Work out the finished part from the listing and answer in its coordinate system (mm). A direction names the side the tool comes from. Coordinates: 2 decimals unless noted, no trailing zeros. Write each loop counter-clockwise with the first axis right and the second up, starting at its lowest first coordinate (ties: lowest second). Pieces come first, ordered by that corner, then holes. Notation, with made-up numbers: M 25,65.25 L 57,65.25 A18 cw 57,81.25 Z; hole C -31,-27.75 d1. An arc over 180 degrees is marked long. Answer as CSV lines item,"result". Start each with the question number.
(1) The mould has two halves that part along Y. Classify faces 6 (the cylindrical face through (36.444, 55.404, 6.409)), 7 (the flat face through (16, 1, 0)), 8 (the cylindrical face through (36.36, -55.38, 6.41)), 9 (the cylindrical face through (-48.234, 45.511, 6.409)): released by +Y, released by -Y, zero draft, split by the parting line, or undercut.
(2) Find the intervals of material crossed by L1, parallel to Y at x = -53.5, z = 11.75; L2, parallel to X at y = -65, z = 8.25; L3, parallel to X at y = 56, z = 9, in increasing order. Write a range as [from, to].
(3) For faces 1 (the flat face through (-17.42, -70, 6.41)), 2 (the flat face through (0, 0, 2)), 3 (the cylindrical face through (-29.78, -59.18, 6.41)), 4 (the flat face through (51.909, -50.084, 6.409)), 5 (the flat face through (-51.909, 50.084, 6.409)), determine the directions among +Z, -Z, +X, -X, +Y, -Y from which every point of the face is accessible in a straight line to the end or side of a thin tool.
(4) A cutting plane is placed at A-A on x = 0. Give the vertices of the cut face in (y, z).
(5) A cutting plane is placed at B-B on z = -3. Give the vertices of the cut face in (x, y), then the cut area to 3 significant figures.
(6) Flat-ended cylindrical pins translate along their axes: P1, Ø3, axis at x = -21, y = 3, coming from the +Z side; P2, Ø2, axis at y = 0, z = 8.5, coming from the -X side; P3, Ø0.9, axis at x = 5, y = -7.5, coming from the -Z side; P4, Ø1, axis at y = -17.5, z = -1.5, coming from the +X side. Find the tip coordinate at first contact, or state that the pin passes through.
from build123d import *

# Parameters (mm, degrees)
F0_R     = 62.5
F0_R_2   = 12.7
F0_R_3   = 1.5
F0_R_4   = 4
F1_DEPTH = 3
F2_DEPTH = 13
F3_DEPTH = 9.5
F4_DEPTH = 2


with BuildPart() as f1:
    # F0 (on Top) → F1 (new body)
    with BuildSketch(Plane.XY):
        Circle(F0_R)
        Circle(F0_R_2, mode=Mode.SUBTRACT)
        Circle(F0_R_2)
        with Locations((-4.75, -8.227241)):
            Circle(F0_R_3, mode=Mode.SUBTRACT)
        with Locations((4.75, -8.227241)):
            Circle(F0_R_3, mode=Mode.SUBTRACT)
        with Locations((-9.5, 0)):
            Circle(F0_R_3, mode=Mode.SUBTRACT)
        with Locations((-4.75, 8.227241)):
            Circle(F0_R_3, mode=Mode.SUBTRACT)
        Circle(F0_R_4, mode=Mode.SUBTRACT)
        with Locations((4.75, 8.227241)):
            Circle(F0_R_3, mode=Mode.SUBTRACT)
        with Locations((9.5, 0)):
            Circle(F0_R_3, mode=Mode.SUBTRACT)
        with Locations((9.5, 0)):
            Circle(F0_R_3)
        with Locations((4.75, 8.227241)):
            Circle(F0_R_3)
        with Locations((-4.75, 8.227241)):
            Circle(F0_R_3)
        with Locations((-9.5, 0)):
            Circle(F0_R_3)
        with Locations((-4.75, -8.227241)):
            Circle(F0_R_3)
        with Locations((4.75, -8.227241)):
            Circle(F0_R_3)
    extrude(amount=F1_DEPTH)

    # F0 (on Top) → F2 (join)
    with BuildSketch(Plane.XY):
        with BuildLine():
            Line((69, 5), (74.833148, 5))
            ThreePointArc((74.833148, 5), (73.860581, 13.023613), (72.030257, 20.895981))
            Line((72.030257, 20.895981), (66.548892, 18.900927))
            ThreePointArc((66.548892, 18.900927), (63.490338, 19.034466), (61.42204, 21.291617))
            Line((61.42204, 21.291617), (60.738, 23.171002))
            ThreePointArc((60.738, 23.171002), (60.87154, 26.229556), (63.12869, 28.297853))
            Line((63.12869, 28.297853), (68.610056, 30.292907))
            ThreePointArc((68.610056, 30.292907), (64.951905, 37.5), (60.539455, 44.271598))
            Line((60.539455, 44.271598), (56.071005, 40.522123))
            ThreePointArc((56.071005, 40.522123), (53.151231, 39.601522), (50.435676, 41.01515))
            Line((50.435676, 41.01515), (49.150101, 42.547239))
            ThreePointArc((49.150101, 42.547239), (48.2295, 45.467012), (49.643129, 48.182567))
            Line((49.643129, 48.182567), (54.111579, 51.932042))
            ThreePointArc((54.111579, 51.932042), (48.209071, 57.453333), (41.746701, 62.307407))
            Line((41.746701, 62.307407), (38.830127, 57.255753))
            ThreePointArc((38.830127, 57.255753), (36.401302, 55.39205), (33.366025, 55.791651))
            Line((33.366025, 55.791651), (31.633975, 56.791651))
            ThreePointArc((31.633975, 56.791651), (29.770271, 59.220477), (30.169873, 62.255753))
            Line((30.169873, 62.255753), (33.086447, 67.307407))
            ThreePointArc((33.086447, 67.307407), (25.651511, 70.476947), (17.918678, 72.828023))
            Line((17.918678, 72.828023), (16.905763, 67.083494))
            ThreePointArc((16.905763, 67.083494), (15.260838, 64.501479), (12.271939, 63.838856))
            Line((12.271939, 63.838856), (10.302324, 64.186152))
            ThreePointArc((10.302324, 64.186152), (7.720308, 65.831077), (7.057685, 68.819976))
            Line((7.057685, 68.819976), (8.070601, 74.564505))
            ThreePointArc((8.070601, 74.564505), (0, 75), (-8.070601, 74.564505))
            Line((-8.070601, 74.564505), (-7.057685, 68.819976))
            ThreePointArc((-7.057685, 68.819976), (-7.720308, 65.831077), (-10.302324, 64.186152))
            Line((-10.302324, 64.186152), (-12.271939, 63.838856))
            ThreePointArc((-12.271939, 63.838856), (-15.260838, 64.501479), (-16.905763, 67.083494))
            Line((-16.905763, 67.083494), (-17.918678, 72.828023))
            ThreePointArc((-17.918678, 72.828023), (-25.651511, 70.476947), (-33.086447, 67.307407))
            Line((-33.086447, 67.307407), (-30.169873, 62.255753))
            ThreePointArc((-30.169873, 62.255753), (-29.770271, 59.220477), (-31.633975, 56.791651))
            Line((-31.633975, 56.791651), (-33.366025, 55.791651))
            ThreePointArc((-33.366025, 55.791651), (-36.401302, 55.39205), (-38.830127, 57.255753))
            Line((-38.830127, 57.255753), (-41.746701, 62.307407))
            ThreePointArc((-41.746701, 62.307407), (-48.209071, 57.453333), (-54.111579, 51.932042))
            Line((-54.111579, 51.932042), (-49.643129, 48.182567))
            ThreePointArc((-49.643129, 48.182567), (-48.2295, 45.467012), (-49.150101, 42.547239))
            Line((-49.150101, 42.547239), (-50.435676, 41.01515))
            ThreePointArc((-50.435676, 41.01515), (-53.151231, 39.601522), (-56.071005, 40.522123))
            Line((-56.071005, 40.522123), (-60.539455, 44.271598))
            ThreePointArc((-60.539455, 44.271598), (-64.951905, 37.5), (-68.610056, 30.292907))
            Line((-68.610056, 30.292907), (-63.12869, 28.297853))
            ThreePointArc((-63.12869, 28.297853), (-60.87154, 26.229556), (-60.738, 23.171002))
            Line((-60.738, 23.171002), (-61.42204, 21.291617))
            ThreePointArc((-61.42204, 21.291617), (-63.490338, 19.034466), (-66.548892, 18.900927))
            Line((-66.548892, 18.900927), (-72.030257, 20.895981))
            ThreePointArc((-72.030257, 20.895981), (-73.860581, 13.023613), (-74.833148, 5))
            Line((-74.833148, 5), (-69, 5))
            ThreePointArc((-69, 5), (-66.171573, 3.828427), (-65, 1))
            Line((-65, 1), (-65, -1))
            ThreePointArc((-65, -1), (-66.171573, -3.828427), (-69, -5))
            Line((-69, -5), (-74.833148, -5))
            ThreePointArc((-74.833148, -5), (-73.860581, -13.023613), (-72.030257, -20.895981))
            Line((-72.030257, -20.895981), (-66.548892, -18.900927))
            ThreePointArc((-66.548892, -18.900927), (-63.490338, -19.034466), (-61.42204, -21.291617))
            Line((-61.42204, -21.291617), (-60.738, -23.171002))
            ThreePointArc((-60.738, -23.171002), (-60.87154, -26.229556), (-63.12869, -28.297853))
            Line((-63.12869, -28.297853), (-68.610056, -30.292907))
            ThreePointArc((-68.610056, -30.292907), (-64.951905, -37.5), (-60.539455, -44.271598))
            Line((-60.539455, -44.271598), (-56.071005, -40.522123))
            ThreePointArc((-56.071005, -40.522123), (-53.151231, -39.601522), (-50.435676, -41.01515))
            Line((-50.435676, -41.01515), (-49.150101, -42.547239))
            ThreePointArc((-49.150101, -42.547239), (-48.2295, -45.467012), (-49.643129, -48.182567))
            Line((-49.643129, -48.182567), (-54.111579, -51.932042))
            ThreePointArc((-54.111579, -51.932042), (-48.209071, -57.453333), (-41.746701, -62.307407))
            Line((-41.746701, -62.307407), (-38.830127, -57.255753))
            ThreePointArc((-38.830127, -57.255753), (-36.401302, -55.39205), (-33.366025, -55.791651))
            Line((-33.366025, -55.791651), (-31.633975, -56.791651))
            ThreePointArc((-31.633975, -56.791651), (-29.770271, -59.220477), (-30.169873, -62.255753))
            Line((-30.169873, -62.255753), (-33.086447, -67.307407))
            ThreePointArc((-33.086447, -67.307407), (-25.651511, -70.476947), (-17.918678, -72.828023))
            Line((-17.918678, -72.828023), (-16.905763, -67.083494))
            ThreePointArc((-16.905763, -67.083494), (-15.260838, -64.501479), (-12.271939, -63.838856))
            Line((-12.271939, -63.838856), (-10.302324, -64.186152))
            ThreePointArc((-10.302324, -64.186152), (-7.720308, -65.831077), (-7.057685, -68.819976))
            Line((-7.057685, -68.819976), (-8.070601, -74.564505))
            ThreePointArc((-8.070601, -74.564505), (0, -75), (8.070601, -74.564505))
            Line((8.070601, -74.564505), (7.057685, -68.819976))
            ThreePointArc((7.057685, -68.819976), (7.720308, -65.831077), (10.302324, -64.186152))
            Line((10.302324, -64.186152), (12.271939, -63.838856))
            ThreePointArc((12.271939, -63.838856), (15.260838, -64.501479), (16.905763, -67.083494))
            Line((16.905763, -67.083494), (17.918678, -72.828023))
            ThreePointArc((17.918678, -72.828023), (25.651511, -70.476947), (33.086447, -67.307407))
            Line((33.086447, -67.307407), (30.169873, -62.255753))
            ThreePointArc((30.169873, -62.255753), (29.770271, -59.220477), (31.633975, -56.791651))
            Line((31.633975, -56.791651), (33.366025, -55.791651))
            ThreePointArc((33.366025, -55.791651), (36.401302, -55.39205), (38.830127, -57.255753))
            Line((38.830127, -57.255753), (41.746701, -62.307407))
            ThreePointArc((41.746701, -62.307407), (48.209071, -57.453333), (54.111579, -51.932042))
            Line((54.111579, -51.932042), (49.643129, -48.182567))
            ThreePointArc((49.643129, -48.182567), (48.2295, -45.467012), (49.150101, -42.547239))
            Line((49.150101, -42.547239), (50.435676, -41.01515))
            ThreePointArc((50.435676, -41.01515), (53.151231, -39.601522), (56.071005, -40.522123))
            Line((56.071005, -40.522123), (60.539455, -44.271598))
            ThreePointArc((60.539455, -44.271598), (64.951905, -37.5), (68.610056, -30.292907))
            Line((68.610056, -30.292907), (63.12869, -28.297853))
            ThreePointArc((63.12869, -28.297853), (60.87154, -26.229556), (60.738, -23.171002))
            Line((60.738, -23.171002), (61.42204, -21.291617))
            ThreePointArc((61.42204, -21.291617), (63.490338, -19.034466), (66.548892, -18.900927))
            Line((66.548892, -18.900927), (72.030257, -20.895981))
            ThreePointArc((72.030257, -20.895981), (73.860581, -13.023613), (74.833148, -5))
            Line((74.833148, -5), (69, -5))
            ThreePointArc((69, -5), (66.171573, -3.828427), (65, -1))
            Line((65, -1), (65, 1))
            ThreePointArc((65, 1), (66.171573, 3.828427), (69, 5))
        make_face()
        Circle(F0_R, mode=Mode.SUBTRACT)
    extrude(amount=F2_DEPTH)

    # F0 (on Top) → F3 (join)
    with BuildSketch(Plane.XY):
        Circle(F0_R_2)
        with Locations((-4.75, -8.227241)):
            Circle(F0_R_3, mode=Mode.SUBTRACT)
        with Locations((4.75, -8.227241)):
            Circle(F0_R_3, mode=Mode.SUBTRACT)
        with Locations((-9.5, 0)):
            Circle(F0_R_3, mode=Mode.SUBTRACT)
        with Locations((-4.75, 8.227241)):
            Circle(F0_R_3, mode=Mode.SUBTRACT)
        Circle(F0_R_4, mode=Mode.SUBTRACT)
        with Locations((4.75, 8.227241)):
            Circle(F0_R_3, mode=Mode.SUBTRACT)
        with Locations((9.5, 0)):
            Circle(F0_R_3, mode=Mode.SUBTRACT)
        with Locations((-4.75, 8.227241)):
            Circle(F0_R_3)
        with Locations((9.5, 0)):
            Circle(F0_R_3)
        with Locations((-4.75, -8.227241)):
            Circle(F0_R_3)
    extrude(amount=-F3_DEPTH)

    # F0 (on Top) → F4 (join)
    with BuildSketch(Plane.XY):
        Circle(F0_R_4)
    extrude(amount=F4_DEPTH)


solid = f1.part
Here are the results:
1,face 6,"released by +Y"
1,face 7,"zero draft"
1,face 8,"released by -Y"
1,face 9,"undercut"
2,L1,"y = [-52.56, -51.42], [-39.59, -32.31], [32.31, 39.59], [51.42, 52.56]"
2,L2,"x = [-31.75, -15.84], [-8.5, 8.5], [15.84, 31.75]"
2,L3,"x = [-49.89, -37.69], [-33.01, -27.75], [27.75, 33.01], [37.69, 49.89]"
3,face 1,"+Z, -Z, -Y"
3,face 2,"+Z"
3,face 3,"+Z, -Z"
3,face 4,"+Z, -Z, +X"
3,face 5,"+Z, -Z, -X"
4,outline,"M -75,0 L -12.7,0 L -12.7,-9.5 L -4,-9.5 L -4,0 L 4,0 L 4,-9.5 L 12.7,-9.5 L 12.7,0 L 75,0 L 75,13 L 62.5,13 L 62.5,3 L 4,3 L 4,2 L -4,2 L -4,3 L -62.5,3 L -62.5,13 L -75,13 Z"
5,outline,"C 0,0 d25.4; hole C -9.5,0 d3; hole C 0,0 d8; hole C 4.75,-8.23 d3; hole C 4.75,8.23 d3"
5,area,"435 mm^2"
6,P1,"stops at z = 3"
6,P2,"stops at x = -65"
6,P3,"stops at z = 0"
6,P4,"passes through"
